from build123d import *

# Parameters (mm, degrees)
SKETCH_2_R          = 1.75
EXTRUDE_1_DEPTH     = 4
SKETCH_3_R          = 2.4
SKETCH_3_R_2        = 1.3
CUT_EXTRUDE_1_DEPTH = 38.089795808


with BuildPart() as part:
    # 草图2 → 凸台-拉伸1 (new body)
    with BuildSketch(Plane(origin=(0, 0, 0), x_dir=(1, 0, 0), z_dir=(0, 1, 0))):
        with BuildLine():
            Line((30.75, 4.085109489), (11.378927035, 4.085109489))
            ThreePointArc((11.378927035, 4.085109489), (-12.09, 0), (11.378927035, -4.085109489))
            Line((11.378927035, -4.085109489), (30.75, -4.085109489))
            ThreePointArc((30.75, -4.085109489), (34.835109489, 0), (30.75, 4.085109489))
        make_face()
        with Locations(Location((30.75, 0, 0), (0, 0, 270))):
            Circle(SKETCH_2_R, mode=Mode.SUBTRACT)
        with Locations(Location((0, 0, 0), (0, 0, 270))):
            Circle(SKETCH_2_R, mode=Mode.SUBTRACT)
    extrude(amount=EXTRUDE_1_DEPTH)

    # 草图3 → 切除-拉伸1 (cut, through all)
    with BuildSketch(Plane(origin=(0, 4, 0), x_dir=(1, 0, 0), z_dir=(0, 1, 0))):
        with Locations(Location((0, 0, 0), (0, 0, 270))):
            Circle(SKETCH_3_R)
        with Locations(Location((4.5, 0, 0), (0, 0, 270))):
            Circle(SKETCH_3_R_2)
        with Locations(Location((-4.5, 0, 0), (0, 0, 270))):
            Circle(SKETCH_3_R_2)
    extrude(amount=-CUT_EXTRUDE_1_DEPTH, mode=Mode.SUBTRACT)


solid = part.part
Input: part model. Units: mm. Frame: model coordinates. A direction names the side the tool comes from. Give positions to 0.01 mm unless a question says otherwise; leave off trailing zeros. Order: outer loops, then holes, each group sorted by start corner. A loop starts at its lowest first (then second) coordinate and runs counter-clockwise, first axis right, second up. Notation, with made-up numbers: (41.25, -31) - (53.25, -31) arc R20 cw to (53.25, -13) - close; hole circle Ø2 at (9, 71). An arc over 180 degrees is marked (long way). Write each question's results on one line, items separated by ' | '.
Item 1: Section A-A (x = 0). Return loops of the section in (y, z), and give its area (3 significant figures).
A:
outline: (0, -12.09) - (4, -12.09) - (4, -2.4) - (0, -2.4) - close; (0, 2.4) - (4, 2.4) - (4, 12.09) - (0, 12.09) - close | area: 77.5 mm^2
Item 2: Section D-D (x = 12). Return loops of the section in (y, z), and give its area (3 significant figures).
A:
outline: (0, -4.09) - (4, -4.09) - (4, 4.09) - (0, 4.09) - close | area: 32.7 mm^2
Item 3: Contact query for flat-ended pins moving along their axis: pin 1 Ø1.5 at (x, y) = (4, 3.5) entering from -Z (3 decimals); pin 2 Ø2 at (x, y) = (19.5, 1.5) entering from -Z. Output: stop coordinate, or through.
A:
pin 1: stops at z = -11.645 | pin 2: stops at z = -4.09
Item 4: Section B-B (y = 2.1). Return loops of the section in (x, z), and give its area (3 significant figures).
A:
outline: (11.38, -4.09) - (30.75, -4.09) arc R4.09 ccw to (30.75, 4.09) - (11.38, 4.09) arc R12.09 ccw (long way) to start; hole circle Ø2.6 at (-4.5, 0); hole circle Ø4.8 at (0, 0); hole circle Ø2.6 at (4.5, 0); hole circle Ø3.5 at (30.75, 0) | area: 601 mm^2
Item 5: Section C-C (z = 0). Return loops of the section in (x, y).
A:
outline: (-12.09, 0) - (-5.8, 0) - (-5.8, 4) - (-12.09, 4) - close; (-3.2, 0) - (-2.4, 0) - (-2.4, 4) - (-3.2, 4) - close; (2.4, 0) - (3.2, 0) - (3.2, 4) - (2.4, 4) - close; (5.8, 0) - (29, 0) - (29, 4) - (5.8, 4) - close; (32.5, 0) - (34.84, 0) - (34.84, 4) - (32.5, 4) - close
Item 6: Access query for faces 1 (the flat face through (21, 2, -4.085)), 2 (the flat face through (21, 2, 4.085)), 3 (the cylindrical face through (3.23, 2.03, -0.28)). Directions: +Z, -Z, +X, -X, +Y, -Y. A direction counts if a zero-diameter tool reaches every point of the face in a straight line with its end or side. Return the directions, or none.
A:
face 1: -Z, +X, +Y, -Y | face 2: +Z, +X, +Y, -Y | face 3: +Y, -Y
Item 7: Material intervals for line 1 along X through (y, z) = (2.45, 0); line 2 along Z through (x, y) = (1, 0.8); line 3 along Z through (x, y) = (5.5, 2.7), sorted ascending.
A:
line 1: x = -12.09 to -5.8, -3.2 to -2.4, 2.4 to 3.2, 5.8 to 29, 32.5 to 34.84 | line 2: z = -12.05 to -2.18, 2.18 to 12.05 | line 3: z = -10.77 to -0.83, 0.83 to 10.77
